Here's the drawing with two shaded views (mm, measured from the low corner). I have some questions. A direction names the side the tool comes from. Coordinates: 2 decimals unless noted, no trailing zeros. Loops run counter-clockwise (first coordinate to the right, second up) from the corner with the lowest first, then second, coordinate; pieces in that order, holes last. Notation, with made-up numbers: (-33.75, -19) -> (-20.75, -19) arc R19 ccw to (-20.75, 1) -> close; hole circle Ø9 at (41, 12.5). An arc over 180 degrees is marked (long way). Use CSV: the item, a comma, the result in double quotes. Start each with the question number.
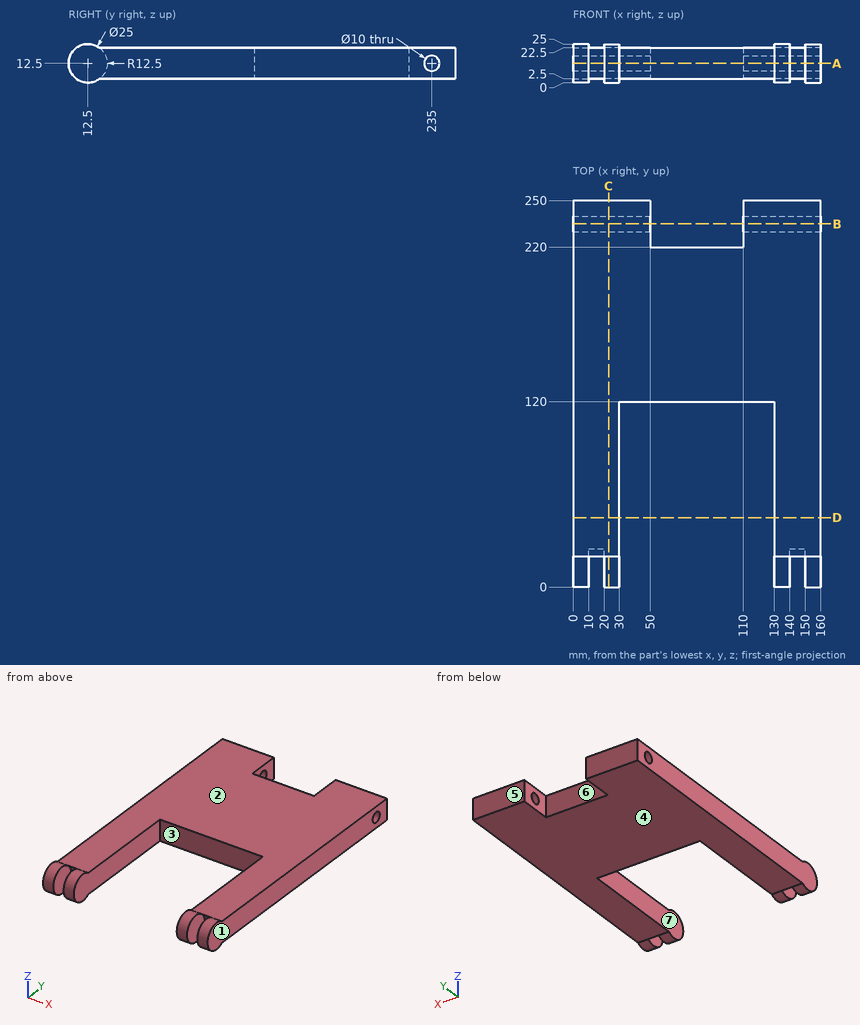
1) Thinking about a two-plate mould opening in X: for the marked faces 1, 2 and 3, which applies, pulls with the +X half, pulls with the -X half, needs draft (parallel to the pull), parting line crosses it, or undercut?
2) I want a section at B-B, the plane y = 235. Please give me the cut outline in (x, z), plus the area to 3 significant figures.
3) For P1, Ø6, axis at x = 134.5, y = 59, coming from the +Z side; P2, Ø12, axis at x = 67, z = 7.5, coming from the -Y side; P3, Ø12, axis at x = 59, y = 173.5, coming from the -Z side, each with a flat end and sliding along its axis, tell me the tip position at first contact or that it passes through.
4) I want a section at A-A, the plane z = 12.5. Please give me the cut outline in (x, y), plus the area to 3 significant figures.
5) I want a section at D-D, the plane y = 45. Please give me the cut outline in (x, z).
6) Please list where these lines run through material, in increasing order: L1, parallel to X at y = 10, z = 16; L2, parallel to Y at x = 36, z = 12.5; L3, parallel to X at y = 66, z = 20.5. Write a range as [from, to].
7) I want a section at C-C, the plane x = 23. Please give me the cut outline in (y, z), plus the area to 3 significant figures.
8) Which directions (+Z, -Z, +X, -X, +Y, -Y) give clear straight access to the entire face, cutting with the end or side of a thin tool? Please do the marked faces 4, 5, 6 and 7.
Return value:
1,face 1,"pulls with the +X half"
1,face 2,"needs draft"
1,face 3,"undercut"
2,outline,"(0, 2.5) -> (50, 2.5) -> (50, 7.5) -> (0, 7.5) -> close; (0, 17.5) -> (50, 17.5) -> (50, 22.5) -> (0, 22.5) -> close; (110, 2.5) -> (160, 2.5) -> (160, 7.5) -> (110, 7.5) -> close; (110, 17.5) -> (160, 17.5) -> (160, 22.5) -> (110, 22.5) -> close"
2,area,"1,000 mm²"
3,P1,"stops at z = 22.5"
3,P2,"stops at y = 120"
3,P3,"stops at z = 2.5"
4,outline,"(0, 0) -> (10, 0) -> (10, 25) -> (20, 25) -> (20, 0) -> (30, 0) -> (30, 120) -> (130, 120) -> (130, 0) -> (140, 0) -> (140, 25) -> (150, 25) -> (150, 0) -> (160, 0) -> (160, 230) -> (110, 230) -> (110, 220) -> (50, 220) -> (50, 230) -> (0, 230) -> close; (0, 240) -> (50, 240) -> (50, 250) -> (0, 250) -> close; (110, 240) -> (160, 240) -> (160, 250) -> (110, 250) -> close"
4,area,"24,700 mm²"
5,outline,"(0, 2.5) -> (30, 2.5) -> (30, 22.5) -> (0, 22.5) -> close; (130, 2.5) -> (160, 2.5) -> (160, 22.5) -> (130, 22.5) -> close"
6,L1,"x = [0, 10], [20, 30], [130, 140], [150, 160]"
6,L2,"y = [120, 230], [240, 250]"
6,L3,"x = [0, 30], [130, 160]"
7,outline,"(20, 2.5) -> (250, 2.5) -> (250, 22.5) -> (20, 22.5) arc R12.5 ccw (long way) to start; hole circle Ø10 at (235, 12.5)"
7,area,"4,940 mm²"
8,face 4,"-Z, +X, -X, +Y"
8,face 5,"+Z, -Z, +X, -X, +Y"
8,face 6,"+Z, -Z, +Y"
8,face 7,"+Z, -Z, -Y"
